Geometry: final body of the model. Coordinates: model frame, mm. A direction names the side the tool comes from. Give positions to 0.01 mm unless a question says otherwise; leave off trailing zeros. Loops run counter-clockwise (first coordinate to the right, second up) from the corner with the lowest first, then second, coordinate; pieces in that order, holes last. Notation, with made-up numbers: (45, 80.5) -> (68, 80.5) arc R20 ccw to (68, 118.5) -> close; hole circle Ø8 at (56.25, -4.75). An arc over 180 degrees is marked (long way). Answer in a Markdown table with one row per item. Add a question column.
1) Section query B-B (x = 81.5). Return the cut outline in (y, z).
2) Access query for faces 1 (the cylindrical face through (69.58, -12.65, 8.06)), 2 (the flat face through (10, 15, 15)), 3 (the flat face through (100, 0, 0)). Directions: +Z, -Z, +X, -X, +Y, -Y. A direction counts if a zero-diameter tool reaches every point of the face in a straight line with its end or side. Return the directions, or none.
3) Section query D-D (z = 12). Return the cut outline in (x, y), plus the area to 3 significant figures.
4) Draft query along Z for faces 4 (the flat face through (0, 4, 9)), 5 (the cylindrical face through (24.79, 34.168, -7.587)), 6 (the flat face through (20, 0, 0)). Return one class per face: +Z half, -Z half, draft (parallel to the pull), parting line (faces both ways), or undercut.
5) Section query A-A (z = 0). Return the cut outline in (x, y).
6) Line query: line 1 (Y direction, x = 16, z = 0); line 2 (X direction, y = 26.5, z = 10); line 3 (X direction, y = -8, z = 15.5). Output: solid intervals per line, ascending. Write a range as from..to.
7) Section query C-C (y = -26.5). Return the cut outline in (x, z).
8) First-contact query: P1, Ø8, axis at x = 12.5, z = 16, coming from the -Y side; P2, Ø10, axis at y = 14, z = -21, coming from the -X side; P3, Ø3, axis at x = 74, z = -17.5, coming from the +Y side; P4, Ø9, axis at y = 0, z = 0, coming from the -X side. Flat tips, straight axial feed; report the tip coordinate or a pass-through.
```python
from build123d import *

# Parameters (mm, degrees)
SKETCH_2_R          = 5
CUT_EXTRUDE_1_DEPTH = 20
SKETCH_3_R          = 9
CUT_EXTRUDE_2_DEPTH = 5
CUT_EXTRUDE_2_TAPER = 38.659808254


with BuildPart() as part:
    # Эскиз1 → Повернуть1 (revolve)
    with BuildSketch(Plane.XY, mode=Mode.PRIVATE) as revolve_1_sk:
        Polygon((0, 0), (100, 0), (100, 15), (40, 15), (40, 35), (10, 35), (10, 20), (0, 20), align=None)
    revolve(revolve_1_sk.sketch.rotate(Axis((0, 0, 0), (1, 0, 0)), 90), axis=Axis((0, 0, 0), (1, 0, 0)))

    # Эскиз2 → Вырез-Вытянуть1 (cut)
    with BuildSketch(Plane(origin=(0, 0, 0), x_dir=(0, 0, -1), z_dir=(1, 0, 0))):
        Circle(SKETCH_2_R)
    extrude(amount=CUT_EXTRUDE_1_DEPTH, mode=Mode.SUBTRACT)

    # Эскиз3 → Вырез-Вытянуть2 (cut)
    with BuildSketch(Plane(origin=(0, 0, 0), x_dir=(0, 0, -1), z_dir=(1, 0, 0))):
        Circle(SKETCH_3_R)
    extrude(amount=CUT_EXTRUDE_2_DEPTH, taper=CUT_EXTRUDE_2_TAPER, mode=Mode.SUBTRACT)


solid = part.part
```
Evaluation:
| question | item | result |
|---|---|---|
| 1 | outline | circle Ø30 at (0, 0) |
| 2 | face 1 | +X |
| 2 | face 2 | -X |
| 2 | face 3 | +Z, -Z, +X, +Y, -Y |
| 3 | outline | (0, -16) -> (10, -16) -> (10, -32.88) -> (40, -32.88) -> (40, -9) -> (100, -9) -> (100, 9) -> (40, 9) -> (40, 32.88) -> (10, 32.88) -> (10, 16) -> (0, 16) -> close |
| 3 | area | 3,370 mm² |
| 4 | face 4 | draft |
| 4 | face 5 | parting line |
| 4 | face 6 | undercut |
| 5 | outline | (0, -20) -> (10, -20) -> (10, -35) -> (40, -35) -> (40, -15) -> (100, -15) -> (100, 15) -> (40, 15) -> (40, 35) -> (10, 35) -> (10, 20) -> (0, 20) -> (0, 9) -> (5, 5) -> (20, 5) -> (20, -5) -> (5, -5) -> (0, -9) -> close |
| 6 | line 1 | -35..-5, 5..35 |
| 6 | line 2 | 10..40 |
| 6 | line 3 | 0..40 |
| 7 | outline | (10, -22.86) -> (40, -22.86) -> (40, 22.86) -> (10, 22.86) -> close |
| 8 | P1 | y = -32.88 |
| 8 | P2 | x = 10 |
| 8 | P3 | through |
| 8 | P4 | x = 20 |
